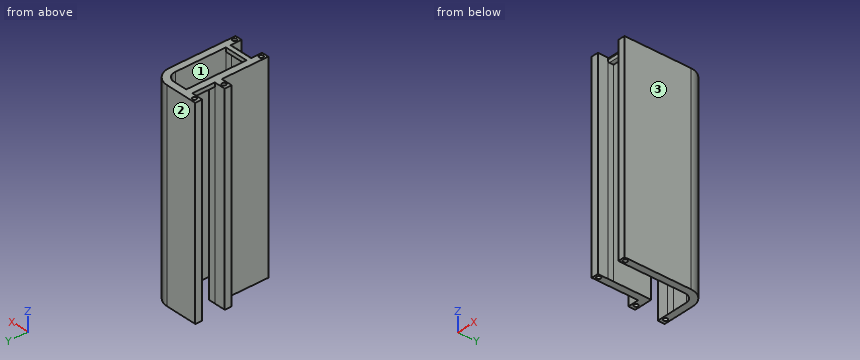
from build123d import *

# Parameters (mm, degrees)
SKETCH_R      = 1.2711848232
PAD_DEPTH     = 127
SKETCH001_W   = 4.436103
SKETCH001_H   = 14.34748
SKETCH001_W_2 = 14.95671
SKETCH001_H_2 = 3.590976
POCKET_DEPTH  = 124.46
FILLET_R      = 0.9906


with BuildPart() as part:
    # Sketch → Pad (new body)
    with BuildSketch(Plane.XY):
        with BuildLine():
            Line((0, 26.6062828995), (-7.1678815, 26.6062828995))
            Line((-7.1678815, 26.6062828995), (-7.1678815, 31.0413108508))
            Line((-7.1678815, 31.0413108508), (13.2402945255, 31.0413108508))
            ThreePointArc((23.8278416124, 20.4537623186), (20.7268209545, 27.9402891709), (13.2402945255, 31.0413108508))
            Line((23.8278416124, 20.4537623186), (23.8278416124, -21.8071686959))
            Line((23.8278416124, -21.8071686959), (19.392813661, -21.8071686959))
            Line((19.392813661, -21.8071686959), (19.392813661, -15.4126492598))
            Line((19.392813661, -15.4126492598), (4.4350279514, -15.4126492598))
            Line((4.4350279514, -15.4126492598), (4.4350279514, -21.7800391169))
            Line((4.4350279514, -21.7800391169), (0, -21.7800391169))
            Line((0, 7.8389965784), (0, -21.7800391169))
            Line((-7.1678815, 7.8389965784), (0, 7.8389965784))
            Line((-7.1678815, 12.2740245298), (-7.1678815, 7.8389965784))
            Line((0, 12.2740245298), (-7.1678815, 12.2740245298))
            Line((0, 26.6062828995), (0, 12.2740245298))
        make_face()
        with Locations((-3.998539, 28.777004)):
            Circle(SKETCH_R, mode=Mode.SUBTRACT)
        with Locations((-3.998539, 10.035677)):
            Circle(SKETCH_R, mode=Mode.SUBTRACT)
        with Locations((2.268514, -19.358597)):
            Circle(SKETCH_R, mode=Mode.SUBTRACT)
        with Locations((21.646236, -19.358597)):
            Circle(SKETCH_R, mode=Mode.SUBTRACT)
        with BuildLine():
            Line((19.392813661, 20.1836425457), (19.392813661, -11.8216736282))
            Line((19.392813661, -11.8216736282), (4.4350279514, -11.8216736282))
            Line((4.4350279514, -11.8216736282), (4.4350279514, 26.5926766868))
            Line((4.4350279514, 26.5926766868), (13.7303997721, 26.5926766868))
            ThreePointArc((19.392813661, 20.1836425457), (17.8554912262, 24.5313130863), (13.7303997721, 26.5926766868))
        make_face(mode=Mode.SUBTRACT)
    extrude(amount=PAD_DEPTH)

    # Sketch001 → Pocket (cut)
    with BuildSketch(Plane.XY):
        with Locations((2.2180515, 19.42961)):
            Rectangle(SKETCH001_W, SKETCH001_H)
        with Locations((11.914458, -13.617161)):
            Rectangle(SKETCH001_W_2, SKETCH001_H_2)
    extrude(amount=POCKET_DEPTH, mode=Mode.SUBTRACT)

    # Fillet
    fillet_edges = [part.edges().sort_by_distance(p)[0] for p in [
        (11.914458, -15.412649, 124.46),
        (11.913921, -15.412649, 127),
    ]]
    fillet(fillet_edges, radius=FILLET_R)


solid = part.part
Read the model definition and answer for the solid it produces. Units are mm, in the model's axes. Face numbers are marked on the shaded views. Round coordinates to 2 decimals unless told otherwise and drop trailing zeros. Write each loop counter-clockwise with the first axis right and the second up, starting at its lowest first coordinate (ties: lowest second). Pieces come first, ordered by that corner, then holes. Notation, with made-up numbers: (-21, 65.25) - (31, 65.25) arc R25 cw to (31, 84.25) - close; hole circle Ø3 at (59.25, -17). An arc over 180 degrees is marked (long way). One line per question, with ' | ' between items. Start each with the question number.
1. Find the intervals of material crossed by probe 1 along X at (y, z) = (1, 121.5); probe 2 along Y at (x, z) = (-1, 112); probe 3 along X at (y, z) = (-19, 97), in increasing order. Write a range as [from, to].
2. Section A-A (y = 14.5) is taken. Determine the outline of the cut face in (x, z).
3. Each of these flat-tipped pins is pushed along its axis until it touches: pin 1 (4 mm diameter, centred on y = -13, z = 65, fed in from -X); pin 2 (7 mm diameter, centred on y = 21.5, z = 63, fed in from -X); pin 3 (4.5 mm diameter, centred on x = 11.5, z = 38.5, fed in from -Y). Where does it stop, or does it pass through?
4. For a pull along X with two mould halves and no side action, classify the marked faces 1, 2 and 3 as +X half, -X half, draft (parallel to the pull), parting line (faces both ways), or undercut.
5. Section D-D (y = 2) is taken. Determine the outline of the cut face in (x, z).
6. Section B-B (x = 11) is taken. Determine the outline of the cut face in (y, z).
7. Section C-C (z = 38.5) is taken. Give the number of separate pieces and of enclosed holes in the cut face, and give its area (3 significant figures).
Filled in:
1) probe 1: [0, 4.44], [19.39, 23.83] | probe 2: [7.84, 12.27], [26.61, 31.04] | probe 3: [0, 1.05], [3.49, 4.44], [19.39, 20.43], [22.87, 23.83]
2) outline: (0, 124.46) - (4.44, 124.46) - (4.44, 127) - (0, 127) - close; (19.39, 0) - (23.83, 0) - (23.83, 127) - (19.39, 127) - close
3) pin 1: x = 0 | pin 2: x = 17.39 | pin 3: y = 26.59
4) face 1: undercut | face 2: draft | face 3: +X half
5) outline: (0, 0) - (4.44, 0) - (4.44, 127) - (0, 127) - close; (19.39, 0) - (23.83, 0) - (23.83, 127) - (19.39, 127) - close
6) outline: (-15.41, 125.45) arc R0.99 ccw to (-14.42, 124.46) - (-11.82, 124.46) - (-11.82, 127) - (-14.42, 127) arc R0.99 ccw to (-15.41, 126.01) - close; (26.59, 0) - (31.04, 0) - (31.04, 127) - (26.59, 127) - close
7) separate pieces: 2 | enclosed holes: 4 | area: 499 mm²
